from build123d import *

# Parameters (mm, degrees)
F1_DEPTH = 152.4
F2_R     = 165.1
F3_DEPTH = 152.4
F4_R     = 165.1
F5_DEPTH = 152.4


with BuildPart() as f1:
    # F0 (on Top) → F1 (new body)
    with BuildSketch(Plane.XY):
        with BuildLine():
            Line((0, 317.5), (0, -317.5))
            Line((0, -317.5), (1778, -317.5))
            Line((1778, -317.5), (1778, -165.1))
            Line((1778, -165.1), (1270, -165.1))
            ThreePointArc((1270, -165.1), (1104.9, 0), (1270, 165.1))
            Line((1270, 165.1), (1778, 165.1))
            Line((1778, 165.1), (1778, 317.5))
            Line((1778, 317.5), (0, 317.5))
        make_face()
    extrude(amount=F1_DEPTH)

    # F2 (on face) → F3 (join)
    with BuildSketch(Plane(origin=(0, 0, 0), x_dir=(0, -1, 0), z_dir=(-1, 0, 0))):
        with BuildLine():
            Line((-317.5, 457.2), (-317.5, 152.4))
            Line((-317.5, 152.4), (317.5, 152.4))
            Line((317.5, 152.4), (317.5, 457.2))
            ThreePointArc((317.5, 457.2), (0, 774.7), (-317.5, 457.2))
        make_face()
        with Locations((0, 457.2)):
            Circle(F2_R, mode=Mode.SUBTRACT)
    extrude(amount=-F3_DEPTH)

    # F4 (on face) → F5 (join)
    with BuildSketch(Plane(origin=(0, 317.5, 0), x_dir=(-1, 0, 0), z_dir=(0, 1, 0))):
        with BuildLine():
            Line((0, -304.8), (0, 0))
            Line((0, 0), (-635, 0))
            Line((-635, 0), (-635, -304.8))
            ThreePointArc((-635, -304.8), (-317.5, -622.3), (0, -304.8))
        make_face()
        with Locations((-317.5, -304.8)):
            Circle(F4_R, mode=Mode.SUBTRACT)
    extrude(amount=-F5_DEPTH)


solid = f1.part
Build history of the part. All positions in model axes, mm. A direction names the side the tool comes from. Round coordinates to 2 decimals unless told otherwise and drop trailing zeros. Write each loop counter-clockwise with the first axis right and the second up, starting at its lowest first coordinate (ties: lowest second). Pieces come first, ordered by that corner, then holes. Notation, with made-up numbers: (-21.75, -31) -> (-6.75, -31) arc R22 ccw to (-6.75, -10) -> close; hole circle Ø1 at (87, 34). An arc over 180 degrees is marked (long way). Use one line per item in the form item = value.
Q1. Band-saw the part on B-B, the plane y = 0. Write the cut outline in (x, z), then the cut area to 3 significant figures.
Conclusion:
outline = (0, 0) -> (1104.9, 0) -> (1104.9, 152.4) -> (152.4, 152.4) -> (152.4, 292.1) -> (0, 292.1) -> close; (0, 622.3) -> (152.4, 622.3) -> (152.4, 774.7) -> (0, 774.7) -> close
area = 213,000 mm²
Q2. Drop flat-ended pins along their axis: P1, Ø5, axis at x = 219, y = -159, coming from the +Z side; P2, Ø1.5, axis at x = 1194, y = -226, coming from the -Z side; P3, Ø8, axis at y = -15, z = 115, coming from the +X side. Give the stop position or say it passes through.
Conclusion:
P1 = 152.4
P2 = 0
P3 = 1106
Q3. Band-saw the part on D-D, the plane z = -401.5. Write the cut outline in (x, y).
Conclusion:
outline = (15.08, 165.1) -> (183.68, 165.1) -> (183.68, 317.5) -> (15.08, 317.5) -> close; (451.32, 165.1) -> (619.92, 165.1) -> (619.92, 317.5) -> (451.32, 317.5) -> close
Q4. Band-saw the part on C-C, the plane z = 125.5. Write the cut outline in (x, y), then the cut area to 3 significant figures.
Conclusion:
outline = (0, -317.5) -> (1778, -317.5) -> (1778, -165.1) -> (1270, -165.1) arc R165.1 cw to (1270, 165.1) -> (1778, 165.1) -> (1778, 317.5) -> (0, 317.5) -> close
area = 918,000 mm²
Q5. Drill centre lines: L1, parallel to Z at x = 317, y = 255; L2, parallel to Z at x = 61, y = 0; L3, parallel to Z at x = 555, y = -132.5. Where is each one in solid material? Low to high.
Conclusion:
L1 = -622.3 to -469.9, -139.7 to 152.4
L2 = 0 to 292.1, 622.3 to 774.7
L3 = 0 to 152.4
Q6. Tool access for faces 4 (the flat face through (181, 165.1, -169)), 5 (the flat face through (1520, 165.1, 75)), 6 (the flat face through (773, 4, 152.4)): list every direction of +Z, -Z, +X, -X, +Y, -Y with a clear straight run to the whole face (end or side of a thin tool).
Conclusion:
face_4 = -Z, +X, -X, -Y
face_5 = +Z, -Z, +X
face_6 = +Z, +X, +Y, -Y
Q7. Band-saw the part on A-A, the plane x = 317.5. Write the cut outline in (y, z).
Conclusion:
outline = (-317.5, 0) -> (165.1, 0) -> (165.1, -139.7) -> (317.5, -139.7) -> (317.5, 152.4) -> (-317.5, 152.4) -> close; (165.1, -622.3) -> (317.5, -622.3) -> (317.5, -469.9) -> (165.1, -469.9) -> close
Q8. Two-plate mould, pull along Y, no slides. Class faces 1 (the flat face through (0, 4, 227)), 2 (the flat face through (564, 317.5, -80)), 3 (the flat face through (1528, -165.1, 75)): released by +Y, released by -Y, zero draft, split by the parting line, or undercut.
Conclusion:
face_1 = zero draft
face_2 = released by +Y
face_3 = undercut
